Verification items for this drawing (mm, ordinates from the low corner). A direction names the side the tool comes from. Coordinates: 2 decimals unless noted, no trailing zeros. Write each loop counter-clockwise with the first axis right and the second up, starting at its lowest first coordinate (ties: lowest second). Pieces come first, ordered by that corner, then holes. Notation, with made-up numbers: (62, -0.75) -> (72, -0.75) arc R18 cw to (72, 26.25) -> close; hole circle Ø7 at (-31, -9). An arc over 180 degrees is marked (long way). Answer as CSV lines item,"result".
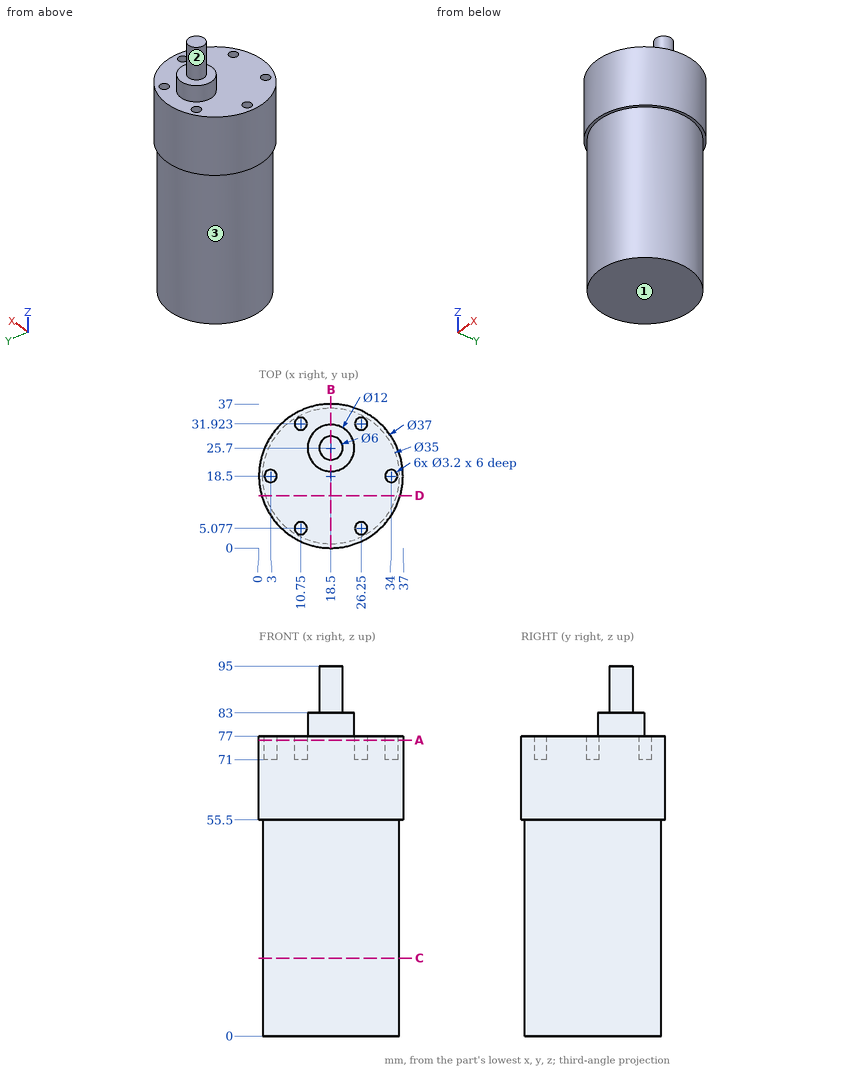
Item 1: Cross-section at D-D, the plane y = 13.5. Record the cut outline in (x, z), plus the area to 3 significant figures.
Responses:
outline,"(0.69, 55.5) -> (1.73, 55.5) -> (1.73, 0) -> (35.27, 0) -> (35.27, 55.5) -> (36.31, 55.5) -> (36.31, 77) -> (0.69, 77) -> close"
area,"2,630 mm2"
Item 2: Cross-section at C-C, the plane z = 20. Record the cut outline in (x, y), plus the area to 3 significant figures.
Responses:
outline,"circle Ø35 at (18.5, 18.5)"
area,"962 mm2"
Item 3: Cross-section at B-B, the plane x = 18.5. Record the cut outline in (y, z), plus the area to 3 significant figures.
Responses:
outline,"(0, 55.5) -> (1, 55.5) -> (1, 0) -> (36, 0) -> (36, 55.5) -> (37, 55.5) -> (37, 77) -> (31.7, 77) -> (31.7, 83) -> (28.7, 83) -> (28.7, 95) -> (22.7, 95) -> (22.7, 83) -> (19.7, 83) -> (19.7, 77) -> (0, 77) -> close"
area,"2,880 mm2"
Item 4: Thickness scan on probe 1 along Y at (x, z) = (26.25, 72.9); probe 2 along X at (y, z) = (18, 74); probe 3 along Z at (x, y) = (6, 23.5). Record the ranges inside material, lowest first.
Responses:
probe 1,"y = 1.7 to 3.48, 6.68 to 30.32, 33.52 to 35.3"
probe 2,"x = 0.01 to 1.48, 4.52 to 32.48, 35.52 to 36.99"
probe 3,"z = 0 to 77"
Item 5: Set-up check for the marked faces 1, 2 and 3: record each of +Z, -Z, +X, -X, +Y, -Y from which the full face is reachable in a straight line by a thin tool's end or side.
Responses:
face 1,"-Z, +X, -X, +Y, -Y"
face 2,"+Z"
face 3,"-Z"
Item 6: Cross-section at A-A, the plane z = 76. Record the cut outline in (x, y).
Responses:
outline,"circle Ø37 at (18.5, 18.5); hole circle Ø3.2 at (3, 18.5); hole circle Ø3.2 at (10.75, 5.08); hole circle Ø3.2 at (10.75, 31.92); hole circle Ø3.2 at (26.25, 5.08); hole circle Ø3.2 at (26.25, 31.92); hole circle Ø3.2 at (34, 18.5)"
Item 7: Depth check by flat-ended pin: pin 1 Ø1 at (x, y) = (23, 24.5) entering from +Z; pin 2 Ø8 at (y, z) = (13.5, 11.5) entering from +X; pin 3 Ø10 at (x, z) = (13, 80) entering from +Y. Enter the tip coordinate at first touch or a pass-through.
Responses:
pin 1,"stops at z = 83"
pin 2,"stops at x = 35.97"
pin 3,"stops at y = 36.94"
